Verification items for this drawing (mm, ordinates from the low corner). A direction names the side the tool comes from. Coordinates: 2 decimals unless noted, no trailing zeros. Order: outer loops, then holes, each group sorted by start corner. A loop starts at its lowest first (then second) coordinate and runs counter-clockwise, first axis right, second up.
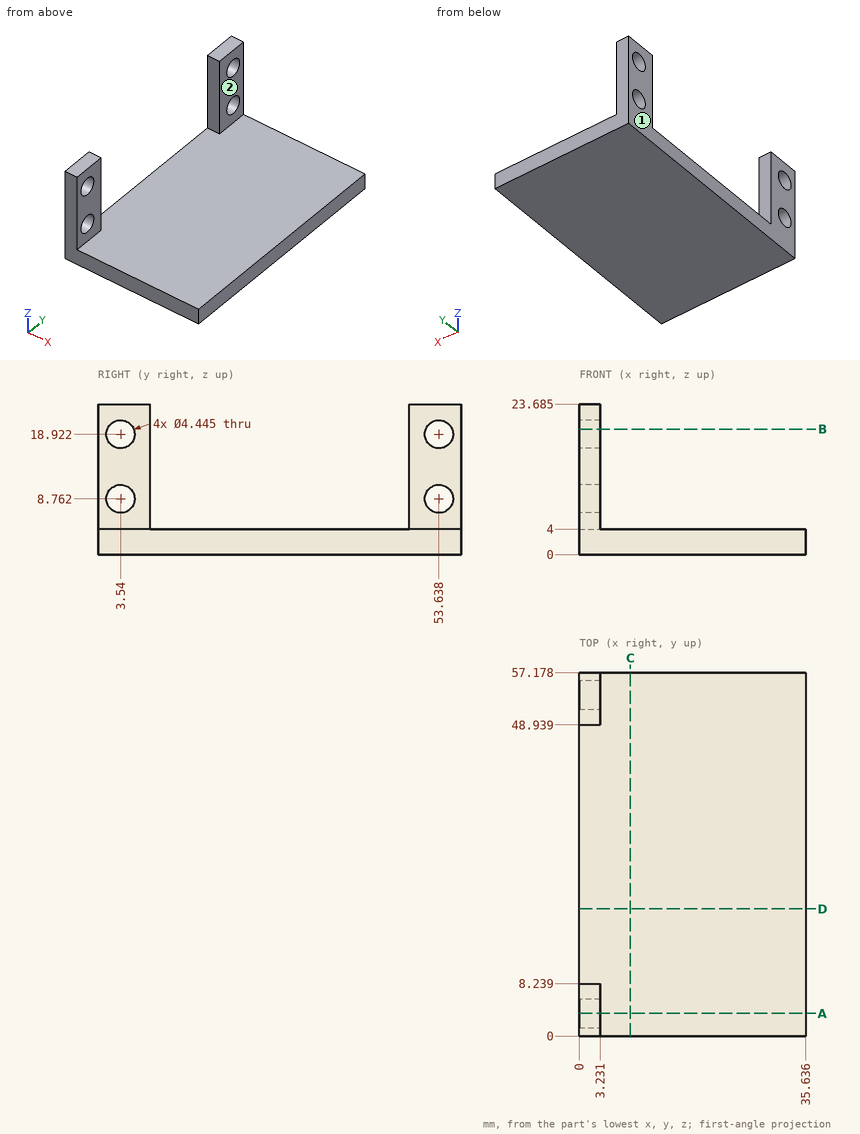
(1) Cross-section at A-A (y = 3.54). Enter the section's corners in (x, z) (1 decimal).
Filled in:
outline: (0, 0) - (35.6, 0) - (35.6, 4) - (3.2, 4) - (3.2, 6.5) - (0, 6.5) - close; (0, 11) - (3.2, 11) - (3.2, 16.7) - (0, 16.7) - close; (0, 21.1) - (3.2, 21.1) - (3.2, 23.7) - (0, 23.7) - close
(2) Thickness scan on probe 1 along Z at (x, y) = (1.75, 3.54) (1 decimal); probe 2 along Z at (x, y) = (4.5, 22.5). Record the ranges inside material, lowest first.
Filled in:
probe 1: z = 0 to 6.5, 11 to 16.7, 21.1 to 23.7
probe 2: z = 0 to 4
(3) Cross-section at D-D (y = 20). Enter the section's corners in (x, z) (1 decimal).
Filled in:
outline: (0, 0) - (35.6, 0) - (35.6, 4) - (0, 4) - close
(4) Cross-section at B-B (z = 19.75). Enter the section's corners in (x, y) (1 decimal).
Filled in:
outline: (0, 0) - (3.2, 0) - (3.2, 1.5) - (0, 1.5) - close; (0, 5.6) - (3.2, 5.6) - (3.2, 8.2) - (0, 8.2) - close; (0, 48.9) - (3.2, 48.9) - (3.2, 51.6) - (0, 51.6) - close; (0, 55.7) - (3.2, 55.7) - (3.2, 57.2) - (0, 57.2) - close
(5) Tool access check on the marked faces 1 and 2. Record the directions out of +Z, -Z, +X, -X, +Y, -Y that give a thin tool (end or side, any length) a straight path to the whole face; none if there is none.
Filled in:
face 1: +Z, -Z, -X, +Y, -Y
face 2: +Z, +X, +Y, -Y
(6) Cross-section at C-C (x = 8). Enter the section's corners in (y, z), and give its area (3 significant figures).
Filled in:
outline: (0, 0) - (57.18, 0) - (57.18, 4) - (0, 4) - close
area: 229 mm2
(7) Go/stop test with flat-tipped pins: P1, Ø6, axis at x = 10.5, y = 47, coming from the -Z side; P2, Ø10, axis at x = 28, y = 30, coming from the +Z side; P3, Ø2.5, axis at y = 53.64, z = 8.76, coming from the +X side; P4, Ø9, axis at y = 5, z = 14.5, coming from the +X side. Record where each tip stops, or that it passes through.
Filled in:
P1: stops at z = 0
P2: stops at z = 4
P3: passes through
P4: stops at x = 3.23
